Autodesk Inventor part; units mm, degrees
ref_plane "YZ Plane" through (0, 0, 0) normal (1, 0, 0) x (0, 1, 0)
ref_plane "XZ Plane" through (0, 0, 0) normal (0, 1, 0) x (-1, 0, 0)
ref_plane "XY Plane" through (0, 0, 0) normal (0, 0, 1) x (1, 0, 0)
sketch "Sketch1" plane through (0, 0, 0) normal (0, 0, 1) x (1, 0, 0)
  circle A0 centre (0, 0) radius 50.8
  circle A1 centre (0, 0) radius 45.72
  circle A2 centre (0, 0) radius 26.67
  circle A3 centre (0, 0) radius 19.05
  circle A4 centre (0, 0) radius 11.43
  line L0 (3.6662, 6.35) -> (7.3323, 0)
  line L1 (7.3323, 0) -> (3.6662, -6.35)
  line L2 (3.6662, -6.35) -> (-3.6662, -6.35)
  line L3 (-3.6662, -6.35) -> (-7.3323, 0)
  line L4 (-7.3323, 0) -> (-3.6662, 6.35)
  line L5 (-3.6662, 6.35) -> (3.6662, 6.35)
  line L6 (0, 0) -> (0, 58.0354)
  line L7 (-2.54, 26.5488) -> (-2.54, 45.6494)
  line L8 (2.54, 26.5488) -> (2.54, 45.6494)
  line L9 (12.7, 23.4521) -> (23.014, 39.5054)
  line L10 (16.9172, 20.6179) -> (27.2549, 36.7081)
  line L11 (24.5372, 10.4506) -> (41.8671, 18.3702)
  line L12 (43.6505, 13.5998) -> (26.0816, 5.571)
  line L13 (26.4637, -3.3108) -> (45.3226, -6.0149)
  line L14 (25.3511, -8.2832) -> (44.3743, -11.0109)
  line L15 (20.2711, -17.3312) -> (34.6746, -29.7992)
  line L16 (16.6011, -20.8733) -> (31.1496, -33.4667)
  line L17 (6.4411, -25.8805) -> (11.8225, -44.165)
  line L18 (1.3677, -26.6349) -> (6.8336, -45.2064)
  line L19 (-6.2201, -25.9345) -> (-11.577, -44.23)
  line L20 (-11.0296, -24.2824) -> (-16.4141, -42.672)
  line L21 (-19.9196, -17.7341) -> (-34.3062, -30.2225)
  line L22 (-22.9299, -13.6202) -> (-37.4507, -26.2252)
  line L23 (-25.9863, -6.0002) -> (-44.8776, -8.7359)
  line L24 (-26.6526, -0.9637) -> (-45.5698, -3.7032)
  line L25 (-25.2585, 8.5613) -> (-42.6471, 16.4785)
  line L26 (-23.177, 13.1954) -> (-40.5558, 21.108)
  line L27 (-14.9508, 22.0854) -> (-25.2719, 38.1005)
  line L28 (-10.4794, 24.5249) -> (-20.8849, 40.6711)
  dimension "d2" = 19.05
  dimension "d0" = 101.6
  dimension "d1" = 5.08
  dimension "d3" = 7.62
  dimension "d4" = 22.86
  dimension "d5" = 12.7
  dimension "d6" = 5.08
  dimension "d7" = 2.54
  dimension "d8" = 5.08
  dimension "d9" = 32.72
  dimension "d10" = 10.16
  dimension "d11" = 32.72
  dimension "d12" = 5.08
  dimension "d13" = 7.62
  dimension "d14" = 5.08
  dimension "d15" = 32.72
  dimension "d16" = 8.89
  dimension "d17" = 32.72
  dimension "d18" = 5.08
  dimension "d19" = 5.08
  dimension "d20" = 32.72
  dimension "d21" = 10.16
  dimension "d22" = 5.08
  dimension "d23" = 5.08
  dimension "d24" = 32.72
  dimension "d25" = 7.62
  dimension "d26" = 5.08
  dimension "d27" = 32.72
  dimension "d28" = 8.89
  dimension "d29" = 5.08
  dimension "d30" = 32.72
  dimension "d31" = 7.62
  dimension "d32" = 5.08
  dimension "d33" = 32.72
  dimension "d34" = 9.525
  dimension "d35" = 5.08
  dimension "d36" = 32.72
  dimension "d37" = 8.89
extrude "Extrusion3" add sketch "Sketch1" along normal blind 25.4 contours A1 L8 A2 L6 | L6 A2 L7 A1 | A0 | A2 | A4 | A1 L10 A2 L9 | L28 A2 L27 A1 | A1 L12 A2 L11 | L26 A2 L25 A1 | L24 A2 L23 A1 | A1 L14 A2 L13 | L22 A2 L21 A1 | A1 L16 A2 L15 | L20 A2 L19 A1 | A1 L18 A2 L17
sketch "Sketch3" plane through (0, 0, 25.4) normal (0, 0, 1) x (1, 0, 0)
  circle A0 centre (0, 0) radius 11.43
  circle A1 centre (0, 0) radius 19.05
extrude "Extrusion4" add sketch "Sketch3" against normal blind 2.54
sketch "Sketch4" plane through (0, 0, 22.86) normal (0, 0, -1) x (-1, 0, 0)
  circle A0 centre (0, 0) radius 11.43
  line L0 (-10.4724, 4.5798) -> (-17.0961, 8.404)
  circle A1 centre (0, 0) radius 19.05
  line L1 (-9.2024, 6.7795) -> (-15.8261, 10.6037)
  line L2 (-7.3323, 0) -> (-3.6662, 6.35)
  line L3 (-3.6662, 6.35) -> (-7.3323, 0)
  line L4 (-3.6662, 6.35) -> (-14.3563, 12.5219)
  line L5 (3.6662, 6.35) -> (-3.6662, 6.35)
  line L6 (-3.6662, 6.35) -> (3.6662, 6.35)
  line L7 (-1.27, -11.3592) -> (-1.27, -19.0076)
  line L8 (1.27, -11.3592) -> (1.27, -19.0076)
  line L9 (-3.6662, -6.35) -> (3.6662, -6.35)
  line L10 (-3.6662, -6.35) -> (-14.3563, -12.5219)
  line L11 (3.6662, -6.35) -> (14.3563, -12.5219)
  line L12 (3.6662, 6.35) -> (14.3563, 12.5219)
  line L13 (-3.6662, -6.35) -> (-7.3323, 0)
  line L14 (3.6662, 6.35) -> (7.3323, 0)
  line L15 (7.3323, 0) -> (3.6662, -6.35)
  line L16 (10.4724, -4.5798) -> (17.0961, -8.404)
  line L17 (9.2024, -6.7795) -> (15.8261, -10.6037)
  line L18 (-10.4724, -4.5798) -> (-17.0961, -8.404)
  line L19 (-9.2024, -6.7795) -> (-15.8261, -10.6037)
  line L20 (9.2024, 6.7795) -> (15.8261, 10.6037)
  line L21 (10.4724, 4.5798) -> (17.0961, 8.404)
  line L22 (-3.6662, 6.35) -> (-3.6662, 18.6939)
  line L23 (3.6662, -6.35) -> (3.6662, -18.6939)
  line L24 (3.6662, -6.35) -> (-3.6662, -6.35)
  line L25 (-1.27, 11.3592) -> (-1.27, 19.0076)
  line L26 (1.27, 11.3592) -> (1.27, 19.0076)
  dimension "d57" = 2.54
  dimension "d62" = 2.54
  dimension "d64" = 2.54
  dimension "d66" = 2.54
  dimension "d68" = 2.54
  dimension "d72" = 2.3962
  dimension "d73" = 2.3962
  dimension "d74" = 2.3962
  dimension "d75" = 2.3962
  dimension "d76" = 2.3962
  dimension "d77" = 2.3962
  dimension "d78" = 2.54
extrude "Extrusion5" add sketch "Sketch4" along normal blind 16.51 contours A0 L20 A1 L21 | L16 A1 L17 A0 | A0 L25 A1 L26 | L8 A1 L7 A0 | A0 L0 A1 L1 | L19 A1 L18 A0
equation "\"d11\" = d9"
equation "\"d15\" = d11"
equation "\"d17\" = d9"
equation "\"d20\" = d9"
equation "\"d24\" = d9"
equation "\"d27\" = d9"
equation "\"d30\" = d9"
equation "\"d33\" = d9"
equation "\"d36\" = d9"
properties part number "RobotArm Wheel"
For this review, take the finished solid that the model builds, in its own axes (mm). A direction names the side the tool comes from. Give positions to 0.01 mm unless a question says otherwise; leave off trailing zeros. Write each loop counter-clockwise with the first axis right and the second up, starting at its lowest first coordinate (ties: lowest second). Pieces come first, ordered by that corner, then holes.
Item 1: Take a section at D-D (z = 4.5). Give the number of separate pieces and of enclosed holes in the cut face, and give its area (3 significant figures).
Item 2: Take a section at B-B (y = -39.5). Give the boundary of the cut face in (x, z), and give its area (3 significant figures).
Item 3: Insertion check: P1, Ø9.5, axis at y = 40, z = 18.5, coming from the +X side; P2, Ø2, axis at x = -6, z = 8, coming from the +Y side; P3, Ø2.5, axis at y = 13.5, z = 16.5, coming from the +X side. Each pin has a flat end and moves straight along its axis. Give the tip position at first contact, or say it passes through.
Item 4: Wall thickness on probe 1 along Y at (x, z) = (0, 16); probe 2 along X at (y, z) = (0, 10.5); probe 3 along Y at (x, z) = (39, 12.5): over which ranges is each line inside the solid? List them lowest first.
Item 5: Take a section at C-C (y = 30.5). Give the boundary of the cut face in (x, z) (3 decimals), and give its area (3 significant figures).
Item 6: Machinability: for faces 3 (the face through (-27.01, -23.89, 12.52)), 4 (the face through (13, 8, 6.35)), which of the approach directions +Z, -Z, +X, -X, +Y, -Y give a long, thin tool a straight path to every point of the face, cutting with its end or side? Answer none if there is none.
Item 7: The part is to be moulded in two halves that separate along X. For faces 1 (the face through (-15.609, 32.485, 12.522)), 2 (the face through (22, 1, 0)), say which applies: +X half, -X half, draft (parallel to the pull), parting line (faces both ways), or undercut.
Item 8: Take a section at A-A (x = 0). Give the boundary of the cut face in (y, z), and give its area (3 significant figures).
Established:
1. separate pieces: 2
1. enclosed holes: 13
1. area: 3,970 mm2
2. outline: (-31.94, 0) - (-23.02, 0) - (-23.02, 25.4) - (-31.94, 25.4) - close; (-15.49, 0) - (-10.19, 0) - (-10.19, 25.4) - (-15.49, 25.4) - close; (5.15, 0) - (10.45, 0) - (10.45, 25.4) - (5.15, 25.4) - close; (23.02, 0) - (31.94, 0) - (31.94, 25.4) - (23.02, 25.4) - close
2. area: 722 mm2
3. P1: stops at x = 36.58
3. P2: stops at y = 50.55
3. P3: stops at x = 49.3
4. probe 1: y = -50.8 to -45.72, -26.67 to -6.35, 6.35 to 50.8
4. probe 2: x = -50.8 to -45.72, -26.67 to -19.05, -11.43 to -7.33, 7.33 to 11.43, 19.05 to 26.67, 45.72 to 50.8
4. probe 3: y = -32.55 to -23.86, -10.24 to -5.11, 11.47 to 17.06, 23.86 to 32.55
5. outline: (-40.625, 0) - (-34.06, 0) - (-34.06, 25.4) - (-40.625, 25.4) - close; (-20.374, 0) - (-14.33, 0) - (-14.33, 25.4) - (-20.374, 25.4) - close; (-2.54, 0) - (2.54, 0) - (2.54, 25.4) - (-2.54, 25.4) - close; (17.228, 0) - (23.266, 0) - (23.266, 25.4) - (17.228, 25.4) - close; (34.06, 0) - (40.625, 0) - (40.625, 25.4) - (34.06, 25.4) - close
5. area: 769 mm2
6. face 3: +Z, -Z
6. face 4: -Z
7. face 1: undercut
7. face 2: draft
8. outline: (-50.8, 0) - (-45.72, 0) - (-45.72, 25.4) - (-50.8, 25.4) - close; (-26.67, 0) - (-19.05, 0) - (-19.05, 6.35) - (-11.43, 6.35) - (-11.43, 0) - (-6.35, 0) - (-6.35, 25.4) - (-26.67, 25.4) - close; (6.35, 0) - (11.43, 0) - (11.43, 6.35) - (19.05, 6.35) - (19.05, 0) - (50.8, 0) - (50.8, 25.4) - (6.35, 25.4) - close
8. area: 1,680 mm2
